Here's how the part is built. I have some questions about the finished solid (model axes, mm). A direction names the side the tool comes from. Coordinates: 2 decimals unless noted, no trailing zeros. Write each loop counter-clockwise with the first axis right and the second up, starting at its lowest first coordinate (ties: lowest second). Pieces come first, ordered by that corner, then holes.
Item 1: I want a section at C-C (y = 6). Please give me the cut outline in (x, z).
Item 2: I want a section at A-A (z = 0). Please give me the cut outline in (x, y).
Item 3: For faces 4 (the face through (2, 0, 0)), 5 (the face through (0, -10.922, 0)), which set-ups out of +Z, -Z, +X, -X, +Y, -Y let a thin tool reach every point of the face, with its end or its side?
Item 4: If we mould it in two halves opening along Y, with no side actions, what happens to faces 1 (the face through (-0.67, -4.34, -1.62)), 2 (the face through (1.23, -10.11, 0.78)), 3 (the face through (0, 38.976, 0))? For each: pulls with the +Y half, pulls with the -Y half, needs draft (parallel to the pull), parting line crosses it, or undercut.
Item 5: Please list where these lines run through material, in increasing order: line 1 (Z direction, x = -0.1, y = 19); line 2 (Y direction, x = 2.2, z = 0.65); line 3 (X direction, y = 31, z = -2.1).
Item 6: I want a section at B-B (x = 0). Please give me the cut outline in (y, z), and give its area (3 significant figures).
from build123d import *

# Parameters (mm, degrees)
SKETCH1_R           = 2.38125
BOSS_EXTRUDE1_DEPTH = 38.9763
SKETCH2_R           = 1.7526
BOSS_EXTRUDE2_DEPTH = 10.922


with BuildPart() as part:
    # Sketch1 → Boss-Extrude1 (new body)
    with BuildSketch(Plane(origin=(0, 0, 0), x_dir=(1, 0, 0), z_dir=(0, 1, 0))):
        with Locations(Location((0, 0, 0), (0, 0, 270))):
            Circle(SKETCH1_R)
    extrude(amount=BOSS_EXTRUDE1_DEPTH)

    # Sketch2 → Boss-Extrude2 (add)
    with BuildSketch(Plane.XZ):
        with Locations(Location((0, 0, 0), (0, 0, 270))):
            Circle(SKETCH2_R)
    extrude(amount=BOSS_EXTRUDE2_DEPTH)

    # Sketch3 → Cut-Revolve1 (revolve, cut)
    with BuildSketch(Plane(origin=(0, 0, 0), x_dir=(0, 0, -1), z_dir=(1, 0, 0)), mode=Mode.PRIVATE) as cut_revolve1_sk:
        Polygon((1.7526, -8.805333333), (1.27, -10.922), (1.7526, -10.922), align=None)
    revolve(cut_revolve1_sk.sketch.rotate(Axis((0, -10.922, 0), (0, 1, 0)), 180), axis=Axis((0, -10.922, 0), (0, 1, 0)), mode=Mode.SUBTRACT)


solid = part.part
Answer:
1. outline: circle Ø4.76 at (0, 0)
2. outline: (-2.38, 0) - (-1.75, 0) - (-1.75, -8.81) - (-1.27, -10.92) - (1.27, -10.92) - (1.75, -8.81) - (1.75, 0) - (2.38, 0) - (2.38, 38.98) - (-2.38, 38.98) - close
3. face 4: -Y
3. face 5: +Z, -Z, +X, -X, -Y
4. face 1: needs draft
4. face 2: pulls with the -Y half
4. face 3: pulls with the +Y half
5. line 1: z = -2.38 to 2.38
5. line 2: y = 0 to 38.98
5. line 3: x = -1.12 to 1.12
6. outline: (-10.92, -1.27) - (-8.81, -1.75) - (0, -1.75) - (0, -2.38) - (38.98, -2.38) - (38.98, 2.38) - (0, 2.38) - (0, 1.75) - (-8.81, 1.75) - (-10.92, 1.27) - close
6. area: 223 mm2
